The figure shows three views and two pictorial views of one solid part (mm, origin at its lowest corner). Answer the questions. A direction names the side the tool comes from. Give positions to 0.01 mm unless a question says otherwise; leave off trailing zeros. Loops run counter-clockwise (first coordinate to the right, second up) from the corner with the lowest first, then second, coordinate; pieces in that order, holes last. Notation, with made-up numbers: (23.5, 56.5) - (49.5, 56.5) arc R30 cw to (49.5, 79.5) - close; hole circle Ø5 at (22, 65.25). An arc over 180 degrees is marked (long way). Use CSV: the item, a comma, the result in double quotes.
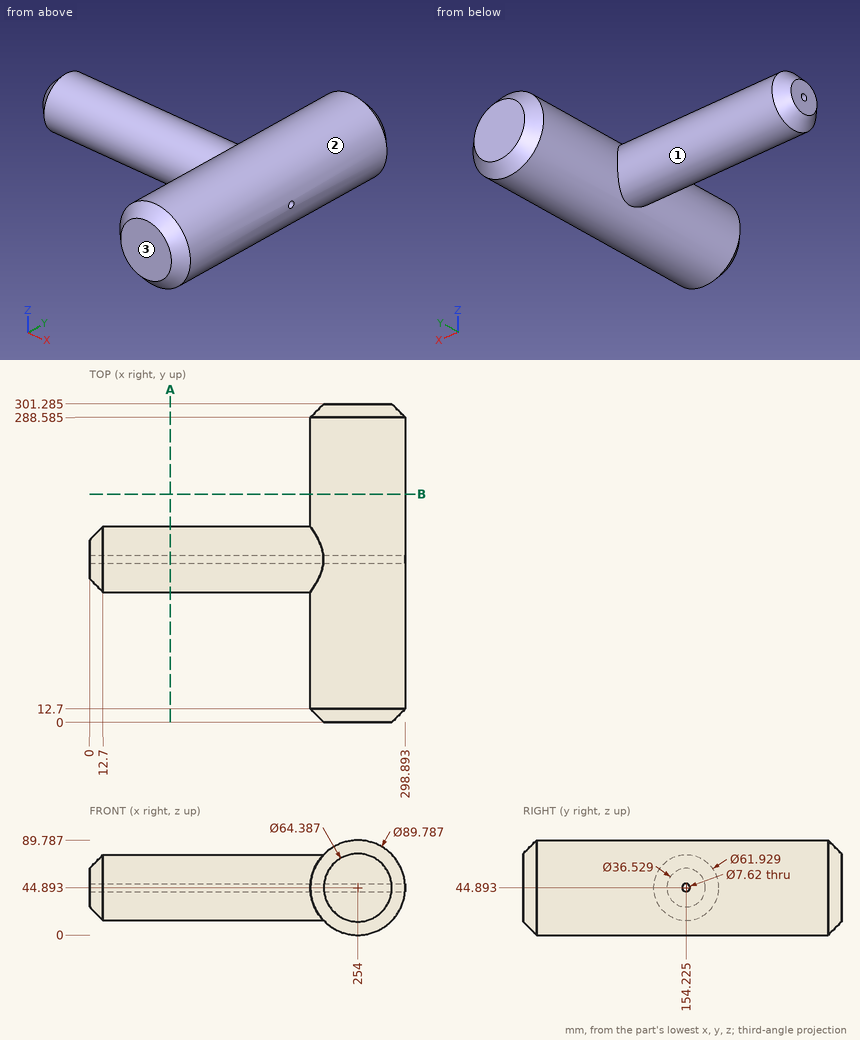
Item 1: Find the intervals of material crossed by line 1 (X direction, y = 201, z = 44) (1 decimal); line 2 (Y direction, x = 48, z = 37) (1 decimal); line 3 (Z direction, x = 241, y = 272) (1 decimal), in increasing order.
Determined:
line 1,"x = 209.1 to 298.9"
line 2,"y = 124.3 to 184.2"
line 3,"z = 1.9 to 87.9"
Item 2: A cutting plane is placed at B-B on y = 216. Determine the outline of the cut face in (x, z), and give its area (3 significant figures).
Determined:
outline,"circle Ø89.79 at (254, 44.89)"
area,"6,330 mm²"
Item 3: Given P1, Ø8, axis at y = 221.5, z = 11, coming from the -X side (1 decimal); P2, Ø1.5, axis at x = 264.5, z = 77.5, coming from the +Y side; P3, Ø6, axis at y = 117.5, z = 32, coming from the +X side, each flat-ended and moving along its own axis, determine where each tip first touches the part or whether it passes through.
Determined:
P1,"stops at x = 220.5"
P2,"stops at y = 299.97"
P3,"stops at x = 297.79"
Item 4: For the marked faces 1, 2 and 3, determine the directions among +Z, -Z, +X, -X, +Y, -Y from which every point of the face is accessible in a straight line to the end or side of a thin tool.
Determined:
face 1,"-X"
face 2,"none"
face 3,"+Z, -Z, +X, -X, -Y"
Item 5: A cutting plane is placed at A-A on x = 76.5. Determine the outline of the cut face in (y, z) (1 decimal), and give its area (3 significant figures).
Determined:
outline,"circle Ø61.9 at (154.2, 44.9); hole circle Ø7.6 at (154.2, 44.9)"
area,"2,970 mm²"
